```python
from build123d import *

# Parameters (mm, degrees)
SKETCH002_W     = 53
SKETCH002_H     = 28
PAD_DEPTH       = 3
SKETCH_R        = 2
POCKET_DEPTH    = 5
SKETCH001_R     = 2
POCKET001_DEPTH = 5
SKETCH003_W     = 53
SKETCH003_H     = 2.5
PAD001_DEPTH    = 20


with BuildPart() as part:
    # Sketch002 → Pad (new body)
    with BuildSketch(Plane.XY):
        with Locations((18.5, -6)):
            Rectangle(SKETCH002_W, SKETCH002_H)
    extrude(amount=PAD_DEPTH)

    # Sketch → Pocket (cut)
    with BuildSketch(Plane.XY):
        Circle(SKETCH_R)
    extrude(amount=POCKET_DEPTH, mode=Mode.SUBTRACT)

    # Sketch001 → Pocket001 (cut)
    with BuildSketch(Plane.XY):
        with Locations((37, 0)):
            Circle(SKETCH001_R)
    extrude(amount=POCKET001_DEPTH, mode=Mode.SUBTRACT)

    # Sketch003 → Pad001 (join)
    with BuildSketch(Plane.XY):
        with Locations((18.5, -18.75)):
            Rectangle(SKETCH003_W, SKETCH003_H)
    extrude(amount=-PAD001_DEPTH)


solid = part.part
```
Geometry: final body of the model. Coordinates: model frame, mm. Coordinates: 2 decimals unless noted, no trailing zeros. Loops run counter-clockwise (first coordinate to the right, second up) from the corner with the lowest first, then second, coordinate; pieces in that order, holes last. Notation, with made-up numbers: (79.25, 72.5) -> (118.25, 72.5) arc R30 cw to (118.25, 105.5) -> close; hole circle Ø5 at (64, -8.5). An arc over 180 degrees is marked (long way). Use a Markdown table: item, result. Add a question column.
(1) Section query B-B, the plane y = 0. Return loops of the section in (x, z).
(2) Section query C-C, the plane x = 24.5. Return loops of the section in (y, z).
(3) Section query A-A, the plane x = 37. Return loops of the section in (y, z), plus the area to 3 significant figures.
(4) Pin query (flat end, axial travel): pin 1 Ø6.5 at (x, y) = (37, 0) entering from -Z; pin 2 Ø4.5 at (x, y) = (0, 0) entering from +Z. Return the tip coordinate at first contact, or that it passes through.
(5) Line query: line 1 along X through (y, z) = (0, 1.9); line 2 along Y through (x, z) = (37, 1.3); line 3 along Y through (x, z) = (10.5, -16.5). Output: solid intervals per line, ascending.
(6) Mould query, pull axis Y, two halves, no side actions, for faces 1 (the flat face through (18, -5, 0)), 2 (the cylindrical face through (35, 0, 1)), 3 (the flat face through (18, -17.5, -10)). Classes: pulls with the +Y half, pulls with the -Y half, needs draft (parallel to the pull), parting line crosses it, or undercut.
(7) Section query D-D, the plane z = -16. Return loops of the section in (x, y).
Answer:
| question | item | result |
|---|---|---|
| 1 | outline | (-8, 0) -> (-2, 0) -> (-2, 3) -> (-8, 3) -> close; (2, 0) -> (35, 0) -> (35, 3) -> (2, 3) -> close; (39, 0) -> (45, 0) -> (45, 3) -> (39, 3) -> close |
| 2 | outline | (-20, -20) -> (-17.5, -20) -> (-17.5, 0) -> (8, 0) -> (8, 3) -> (-20, 3) -> close |
| 3 | outline | (-20, -20) -> (-17.5, -20) -> (-17.5, 0) -> (-2, 0) -> (-2, 3) -> (-20, 3) -> close; (2, 0) -> (8, 0) -> (8, 3) -> (2, 3) -> close |
| 3 | area | 122 mm^2 |
| 4 | pin 1 | stops at z = 0 |
| 4 | pin 2 | stops at z = 3 |
| 5 | line 1 | x = -8 to -2, 2 to 35, 39 to 45 |
| 5 | line 2 | y = -20 to -2, 2 to 8 |
| 5 | line 3 | y = -20 to -17.5 |
| 6 | face 1 | needs draft |
| 6 | face 2 | undercut |
| 6 | face 3 | pulls with the +Y half |
| 7 | outline | (-8, -20) -> (45, -20) -> (45, -17.5) -> (-8, -17.5) -> close |
